Build history of the part. All positions in model axes, mm. A direction names the side the tool comes from. Give positions to 0.01 mm unless a question says otherwise; leave off trailing zeros. Order: outer loops, then holes, each group sorted by start corner. A loop starts at its lowest first (then second) coordinate and runs counter-clockwise, first axis right, second up. Notation, with made-up numbers: (23.25, 55.5) -> (65.25, 55.5) arc R22 cw to (65.25, 61.5) -> close; hole circle Ø8 at (48.25, 61.25). An arc over 180 degrees is marked (long way). Use a Markdown table: item, result. Add a question column.
```python
from build123d import *

# Parameters (mm, degrees)
F1_W     = 65
F1_H     = 65
F2_DEPTH = 720
F3_W     = 1246
F3_H     = 556
F4_DEPTH = 150
F5_W     = 1285
F5_H     = 620
F6_DEPTH = 30


with BuildPart() as f2:
    # F1 (on Top) → F2 (new body, through all)
    with BuildSketch(Plane.XY):
        with Locations((52.5, 557.5)):
            Rectangle(F1_W, F1_H)
        with Locations((1237.5, 62.5)):
            Rectangle(F1_W, F1_H)
        with Locations((1237.5, 557.5)):
            Rectangle(F1_W, F1_H)
        with Locations((52.5, 62.5)):
            Rectangle(F1_W, F1_H)
    extrude(amount=F2_DEPTH)

    # F3 (on offset) → F4 (join)
    with BuildSketch(Plane.XY.offset(720)):
        with Locations((645, 310)):
            Rectangle(F3_W, F3_H)
    extrude(amount=-F4_DEPTH)

    # F5 (on offset) → F6 (join)
    with BuildSketch(Plane.XY.offset(720)):
        with Locations((644.5, 312)):
            Rectangle(F5_W, F5_H)
    extrude(amount=F6_DEPTH)


solid = f2.part
```
(1) Mould opens along X. For faces 4 (the face through (22, 307, 646)), 5 (the face through (52, 63, 0)), 6 (the face through (1268, 307, 646)), 7 (the face through (637, 32, 646)) say: released by +X, released by -X, zero draft, split by the parting line, or undercut.
(2) Wall check: probe 1 along X at (y, z) = (538.5, 393.5); probe 2 along Z at (x, y) = (1099.5, 326.5); probe 3 along Y at (x, z) = (198, 600). Give the ranges that are in metal, low to high.
(3) Band-saw the part on C-C on y = 451.5. Give the cut face in (x, z), plus the area to 3 significant figures.
(4) Band-saw the part on B-B on z = 634. Give the cut face in (x, y), plus the area to 3 significant figures.
(5) Band-saw the part on D-D on x = 1162.5. Give the cut face in (y, z).
(6) Band-saw the part on A-A on z = 431. Give the cut face in (x, y).
(7) Tool access for faces 1 (the face through (1270, 62, 355)), 2 (the face through (1237, 590, 355)), 3 (the face through (20, 557, 355)): list every direction of +Z, -Z, +X, -X, +Y, -Y with a clear straight run to the whole face (end or side of a thin tool).
(8) Pin check, flat tips, straight feed: pin 1 Ø19.5 at (x, z) = (40, 475.5) entering from -Y; pin 2 Ø5 at (x, y) = (977.5, 399.5) entering from -Z; pin 3 Ø19.5 at (y, z) = (559, 472) entering from +X. Stop position of each tip, or through.
Response:
| question | item | result |
|---|---|---|
| 1 | face 4 | released by -X |
| 1 | face 5 | zero draft |
| 1 | face 6 | released by +X |
| 1 | face 7 | undercut |
| 2 | probe 1 | x = 20 to 85, 1205 to 1270 |
| 2 | probe 2 | z = 570 to 750 |
| 2 | probe 3 | y = 32 to 588 |
| 3 | outline | (2, 720) -> (22, 720) -> (22, 570) -> (1268, 570) -> (1268, 720) -> (1287, 720) -> (1287, 750) -> (2, 750) -> close |
| 3 | area | 225,000 mm² |
| 4 | outline | (20, 30) -> (85, 30) -> (85, 32) -> (1205, 32) -> (1205, 30) -> (1270, 30) -> (1270, 95) -> (1268, 95) -> (1268, 525) -> (1270, 525) -> (1270, 590) -> (1205, 590) -> (1205, 588) -> (85, 588) -> (85, 590) -> (20, 590) -> (20, 525) -> (22, 525) -> (22, 95) -> (20, 95) -> close |
| 4 | area | 694,000 mm² |
| 5 | outline | (2, 720) -> (32, 720) -> (32, 570) -> (588, 570) -> (588, 720) -> (622, 720) -> (622, 750) -> (2, 750) -> close |
| 6 | outline | (20, 30) -> (85, 30) -> (85, 95) -> (20, 95) -> close; (20, 525) -> (85, 525) -> (85, 590) -> (20, 590) -> close; (1205, 30) -> (1270, 30) -> (1270, 95) -> (1205, 95) -> close; (1205, 525) -> (1270, 525) -> (1270, 590) -> (1205, 590) -> close |
| 7 | face 1 | -Z, +X, +Y, -Y |
| 7 | face 2 | -Z, +X, -X, +Y |
| 7 | face 3 | -Z, -X, +Y, -Y |
| 8 | pin 1 | stops at y = 30 |
| 8 | pin 2 | stops at z = 570 |
| 8 | pin 3 | stops at x = 1270 |
